Verification items for the finished model (mm, model axes). Face numbers are marked on the shaded views. Coordinates: 2 decimals unless noted, no trailing zeros. Write each loop counter-clockwise with the first axis right and the second up, starting at its lowest first coordinate (ties: lowest second). Pieces come first, ordered by that corner, then holes. Notation, with made-up numbers: M 59.25,-18 L 79.25,-18 A27 ccw 79.25,0 Z; hole C 21,87.5 d5. An arc over 180 degrees is marked long. Answer in a Markdown table with one row per item.
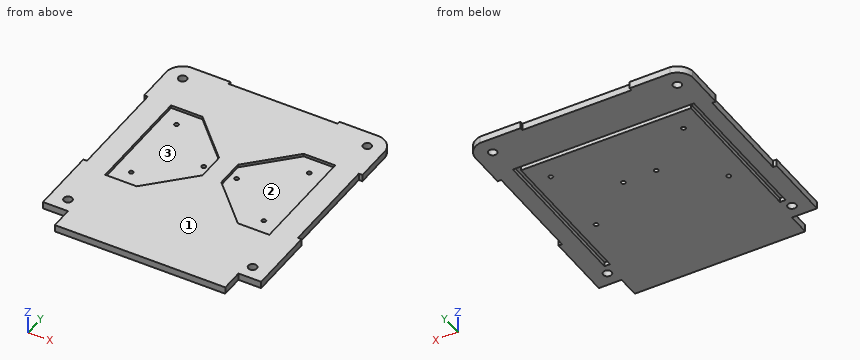
from build123d import *

# Parameters (mm, degrees)
BOSS_EXTRUDE1_DEPTH = 5
CUT_EXTRUDE1_DEPTH  = 2
SKETCH3_R           = 3
CUT_EXTRUDE2_DEPTH  = 42
SKETCH6_W           = 4
SKETCH6_H           = 4
SKETCH6_W_2         = 3.999984741
CUT_EXTRUDE4_DEPTH  = 3
CUT_EXTRUDE5_DEPTH  = 3
SKETCH8_W           = 121.9
SKETCH8_H           = 16
BOSS_EXTRUDE2_DEPTH = 5
SKETCH10_R          = 1.5
CUT_EXTRUDE6_DEPTH  = 10


with BuildPart() as part:
    # Sketch1 → Boss-Extrude1 (new body)
    with BuildSketch(Plane.XY):
        with BuildLine():
            Line((-75.420043945, 42.350021362), (-75.420043945, -31.650009155))
            Line((-75.420043945, -31.650009155), (-78, -31.650009155))
            Line((-78, -31.650009155), (-78, -80.650009155))
            Line((-78, -80.650009155), (78, -80.650009155))
            Line((78, -80.650009155), (78, -31.650009155))
            Line((78, -31.650009155), (75.419921875, -31.650009155))
            Line((75.419921875, -31.650009155), (75.419921875, 42.350021362))
            Line((75.419921875, 42.350021362), (78, 42.350021362))
            Line((78, 42.350021362), (78, 70.650009155))
            ThreePointArc((78, 70.650009155), (74.602310181, 77.252319336), (68, 80.650009155))
            Line((68, 80.650009155), (39, 80.650009155))
            Line((39, 80.650009155), (39, 78.449996948))
            Line((39, 78.449996948), (-39, 78.449996948))
            Line((-39, 78.449996948), (-39, 80.650009155))
            Line((-39, 80.650009155), (-68, 80.650009155))
            ThreePointArc((-68, 80.650009155), (-74.602340698, 77.252349854), (-78, 70.650009155))
            Line((-78, 70.650009155), (-78, 42.350021362))
            Line((-78, 42.350021362), (-75.420043945, 42.350021362))
        make_face()
    extrude(amount=BOSS_EXTRUDE1_DEPTH)

    # Sketch2 → Cut-Extrude1 (cut)
    with BuildSketch(Plane.XY.offset(5)):
        Polygon((-6.739431127, -7.975087618), (-6.739431127, 12.139103822), (-36.191468123, 42.082008102), (-58.691468123, 42.082008102), (-58.691468123, 2.082008102), (-58.691468123, -37.917991898), (-36.191468123, -37.917991898), align=None)
        Polygon((6.739431127, 12.139103822), (36.191468123, 42.082008102), (58.691468123, 42.082008102), (58.691468123, 2.082008102), (58.691468123, -37.917991898), (36.191468123, -37.917991898), (6.739431127, -7.975087618), align=None)
    extrude(amount=-CUT_EXTRUDE1_DEPTH, mode=Mode.SUBTRACT)

    # Sketch3 → Cut-Extrude2 (cut)
    with BuildSketch(Plane.XY.offset(5)):
        with Locations((-66.000082844, 68.650091999)):
            Circle(SKETCH3_R)
        with Locations((65.999919006, 68.649928161)):
            Circle(SKETCH3_R)
        with Locations((-66.000082844, -70.650009155)):
            Circle(SKETCH3_R)
        with Locations((65.999919006, -70.650009155)):
            Circle(SKETCH3_R)
    extrude(amount=-CUT_EXTRUDE2_DEPTH, mode=Mode.SUBTRACT)

    # Sketch6 → Cut-Extrude4 (cut)
    with BuildSketch(Plane(origin=(0, 0, 0), x_dir=(-1, 0, 0), z_dir=(0, 0, -1))):
        with Locations((-61.995116115, -61.665595666)):
            Rectangle(SKETCH6_W, SKETCH6_H)
        with Locations((63.504872442, -61.665595666)):
            Rectangle(SKETCH6_W_2, SKETCH6_H)
    extrude(amount=-CUT_EXTRUDE4_DEPTH, mode=Mode.SUBTRACT)

    # Sketch7 → Cut-Extrude5 (cut)
    with BuildSketch(Plane(origin=(0, 0, 0), x_dir=(-1, 0, 0), z_dir=(0, 0, -1))):
        Polygon((-63.995116115, -59.665595666), (-63.995116115, 47.660531993), (65.504864812, 47.660531993), (65.504864812, -59.665595666), (61.504880071, -59.665595666), (61.504880071, 44.476086648), (-59.995116115, 44.476086648), (-59.995116115, -59.665595666), align=None)
    extrude(amount=-CUT_EXTRUDE5_DEPTH, mode=Mode.SUBTRACT)

    # Sketch8 → Boss-Extrude2 (add)
    with BuildSketch(Plane(origin=(0, 0, 0), x_dir=(-1, 0, 0), z_dir=(0, 0, -1))):
        with Locations((-0.820022175, -88.650009155)):
            Rectangle(SKETCH8_W, SKETCH8_H)
    extrude(amount=-BOSS_EXTRUDE2_DEPTH)

    # Sketch10 → Cut-Extrude6 (cut)
    with BuildSketch(Plane.XY.offset(3)):
        with Locations((-47.441468123, 29.582008102)):
            Circle(SKETCH10_R)
        with Locations((-47.441468123, -25.417991898)):
            Circle(SKETCH10_R)
        with Locations((-11.759431127, 2.082008102)):
            Circle(SKETCH10_R)
        with Locations((11.759431127, 2.082008102)):
            Circle(SKETCH10_R)
        with Locations((47.441468123, -25.417991898)):
            Circle(SKETCH10_R)
        with Locations((47.441468123, 29.582008102)):
            Circle(SKETCH10_R)
    extrude(amount=-CUT_EXTRUDE6_DEPTH, mode=Mode.SUBTRACT)


solid = part.part
1) Sectioned sample at C-C (z = 3.75). Give the number of separate pieces and of enclosed holes in the cut face, then the cut area to 3 significant figures.
Response values:
| item | result |
|---|---|
| separate pieces | 1 |
| enclosed holes | 6 |
| area | 19,800 mm² |
2) Thickness scan on L1, parallel to X at y = -62, z = 1.6; L2, parallel to X at y = -15.5, z = 0.2; L3, parallel to Y at x = 36, z = 2.3. Record the ranges inside material, lowest first. Write a range as [from, to].
Response values:
| item | result |
|---|---|
| L1 | x = [-78, -65.5], [-61.5, 60], [64, 78] |
| L2 | x = [-75.42, -65.5], [-61.5, 60], [64, 75.42] |
| L3 | y = [-96.65, 44.48], [47.66, 78.45] |
3) Sectioned sample at A-A (x = -1). Record the cut outline in (y, z).
Response values:
| item | result |
|---|---|
| outline | M -96.65,0 L 44.48,0 L 44.48,3 L 47.66,3 L 47.66,0 L 78.45,0 L 78.45,5 L -96.65,5 Z |
4) Sectioned sample at D-D (x = 56). Record the cut outline in (y, z).
Response values:
| item | result |
|---|---|
| outline | M -96.65,0 L 44.48,0 L 44.48,3 L 47.66,3 L 47.66,0 L 80.65,0 L 80.65,5 L 42.08,5 L 42.08,3 L -37.92,3 L -37.92,5 L -96.65,5 Z |
5) Sectioned sample at B-B (y = -35.5). Record the cut outline in (x, z).
Response values:
| item | result |
|---|---|
| outline | M -78,0 L -65.5,0 L -65.5,3 L -61.5,3 L -61.5,0 L 60,0 L 60,3 L 64,3 L 64,0 L 78,0 L 78,5 L 58.69,5 L 58.69,3 L 33.81,3 L 33.81,5 L -33.81,5 L -33.81,3 L -58.69,3 L -58.69,5 L -78,5 Z |
6) Release check for a two-part mould opening along X. For the marked faces 1, 2 and 3 record: +X half, -X half, draft (parallel to the pull), parting line (faces both ways), or undercut.
Response values:
| item | result |
|---|---|
| face 1 | draft |
| face 2 | undercut |
| face 3 | undercut |
7) Depth check by flat-ended pin: pin 1 (1.6 mm diameter, centred on y = -1.5, z = 4.5, fed in from +X); pin 2 (1.5 mm diameter, centred on y = -3.5, z = 3, fed in from -X); pin 3 (3 mm diameter, centred on x = -10.5, z = 3.5, fed in from +Y). Enter the tip coordinate at first touch or a pass-through.
Response values:
| item | result |
|---|---|
| pin 1 | stops at x = 75.42 |
| pin 2 | stops at x = -75.42 |
| pin 3 | stops at y = 78.45 |
